Autodesk Inventor part; units mm, degrees
ref_plane "YZ Plane" through (0, 0, 0) normal (1, 0, 0) x (0, 1, 0)
ref_plane "XZ Plane" through (0, 0, 0) normal (0, 1, 0) x (-1, 0, 0)
ref_plane "XY Plane" through (0, 0, 0) normal (0, 0, 1) x (1, 0, 0)
sketch "Sketch1" plane through (0, 0, 0) normal (0, 0, 1) x (1, 0, 0)
  line L0 (-33.82, 21.26) -> (-13.5, 21.26)
  line L1 (-13.5, 21.26) -> (-13.5, 6.02)
  line L2 (-13.5, 6.02) -> (-16.04, 6.02)
  line L3 (-16.04, 6.02) -> (-18.58, 16.18)
  line L4 (-18.58, 16.18) -> (-33.82, 16.18)
  line L5 (-33.82, 16.18) -> (-33.82, 21.26)
  dimension "d0" = 20.32
  dimension "d1" = 15.24
  dimension "d2" = 5.08
  dimension "d3" = 2.54
  dimension "d4" = 15.24
extrude "Extrusion1" add sketch "Sketch1" along normal blind 2.54
ref_plane "Work Plane1" through (0, 0, 1.27) normal (0, 0, 1) x (1, 0, 0)
sketch "Sketch2" plane through (0, 0, 1.27) normal (0, 0, 1) x (1, 0, 0)
  line L0 (-33.82, 18.974) -> (-36.36, 18.974)
  arc A0 (-36.36, 18.974) -> (-35.5534, 12.624) centre (-10.96, 18.974) ccw
  line L1 (-35.5534, 12.624) -> (-33.82, 12.624)
  line L2 (-33.82, 12.624) -> (-33.82, 18.974)
  line L3 (-33.82, 16.18) -> (-33.82, 21.26)
  line L4 (-33.82, 21.26) -> (-13.5, 21.26)
  dimension "d8" = 2.54
  dimension "d9" = 6.35
  dimension "d10" = 25.4
  dimension "d11" = 2.286
revolve "Revolution1" add sketch "Sketch2" angle 360 about axis through (-33.82, 18.974, 1.27) along (-1, 0, 0)
sketch "Sketch3" plane through (0, 0, 1.27) normal (0, 0, 1) x (1, 0, 0)
  line L0 (-16.04, 6.02) -> (-18.58, 6.02)
  line L1 (-18.58, 6.02) -> (-18.58, 18.72)
  line L2 (-18.58, 18.72) -> (-16.04, 18.72)
  line L3 (-16.04, 18.72) -> (-16.04, 6.02)
  line L4 (-13.5, 6.02) -> (-16.04, 6.02)
  dimension "d13" = 12.7
  dimension "d14" = 2.54
extrude "Extrusion2" add sketch "Sketch3" along normal mid plane 1.016
sketch "Sketch4" plane through (-13.5, 6.02, 0) normal (1, 0, 0) x (0, 0, -1)
  line L0 (-2.54, 15.24) -> (-2.54, 0)
  line L1 (0, 15.24) -> (-2.54, 15.24)
  line L2 (-2.54, 0) -> (99.06, 0)
  line L3 (-2.54, 6.35) -> (99.06, 6.35)
  line L4 (99.06, 6.35) -> (99.06, 0)
  dimension "d17" = 6.35
  dimension "d18" = 101.6
extrude "Extrusion3" add sketch "Sketch4" against normal blind 2.54
ref_plane "Work Plane2" through (-13.5, 13.64, 0) normal (0, 1, 0) x (1, 0, 0)
sketch "Sketch5" plane through (-13.5, 13.64, 0) normal (0, 1, 0) x (1, 0, 0)
  circle A0 centre (-1.27, 29.21) radius 2.286
  line L0 (0, 99.06) -> (0, 0)
  line L1 (-20.32, -2.54) -> (0, -2.54)
  dimension "d22" = 4.572
  dimension "d23" = 1.27
  dimension "d24" = 31.75
extrude "Extrusion4" add sketch "Sketch5" against normal blind 8.89
sketch "Sketch6" plane through (-16.04, 12.37, 0) normal (0, 1, 0) x (1, 0, 0)
  arc A0 (0, 27.3092) -> (2.54, 27.3092) centre (1.27, 29.21) ccw
  line L0 (0, 27.3092) -> (0, 0)
  line L1 (2.54, 27.3092) -> (2.54, 0)
  line L2 (1.27, 29.21) -> (-2.54, 29.21)
  line L3 (-2.54, 29.21) -> (-2.54, 27.178)
  line L4 (-2.54, 27.178) -> (1.27, 27.178)
  line L5 (1.27, 27.178) -> (1.27, 29.21)
  line L6 (-2.54, -1.778) -> (-2.54, -0.762)
  dimension "d27" = 2.032
extrude "Extrusion5" add sketch "Sketch6" against normal up to surface (6.35 mm away)
sketch "Sketch7" plane through (-16.04, 6.02, -99.06) normal (0, -1, 0) x (1, 0, 0)
  line L0 (0, 67.9492) -> (0, 0)
  line L1 (2.54, 67.9492) -> (2.54, 0)
  circle A0 centre (1.27, 0) radius 3.81
  circle A1 centre (1.27, 0) radius 1.27 construction
  arc A2 (2.54, 71.7508) -> (-1.016, 69.85) centre (1.27, 69.85) ccw
  dimension "d31" = 7.62
  dimension "d42" = 69.85
extrude "Extrusion6" add sketch "Sketch7" against normal up to surface (6.35 mm away)
sketch "Sketch8" plane through (-14.77, 6.02, -29.21) normal (0, -1, 0) x (1, 0, 0)
  arc A0 (-1.27, -66.2579) -> (1.27, -66.2579) centre (0, -69.85) ccw
hole "Hole1" at (-14.77, 6.02, -99.06) direction (0, 1, 0) diameter 3.81 end through all
sketch "Sketch9" plane through (-13.5, 6.02, 2.54) normal (1, 0, 0) x (0, 0, -1)
  line L0 (29.8492, 6.35) -> (2.54, 6.35)
  line L1 (0, 0) -> (29.8492, 0)
  circle A0 centre (14.8195, 3.175) radius 3.175 construction
  line L2 (0, 15.24) -> (0, 0)
  line L3 (12.7, 4.699) -> (25.4, 4.699)
  line L4 (25.4, 4.699) -> (25.4, 1.651)
  line L5 (25.4, 1.651) -> (12.7, 1.651)
  line L6 (12.7, 1.651) -> (12.7, 4.699)
  circle A1 centre (14.8195, 3.175) radius 1.524 construction
  dimension "d46" = 12.7
  dimension "d47" = 12.7
  dimension "d48" = 3.048
extrude "Extrusion7" cut sketch "Sketch9" against normal blind 1.27
properties part number "lock"
Design review of the part built by this model. Coordinates are the model's own, in mm. A direction names the side the tool comes from. Give positions to 0.01 mm unless a question says otherwise; leave off trailing zeros. Order: outer loops, then holes, each group sorted by start corner. A loop starts at its lowest first (then second) coordinate and runs counter-clockwise, first axis right, second up.
1. Tool access review of faces 4 (the flat face through (-15, 12.37, -69)), 5 (the flat face through (-13.5, 9, -64)), 6 (the flat face through (-15, 6.02, -69)), 7 (the flat face through (-16.04, 9, -13)), 8 (the flat face through (-14.77, 9, -16)): name each direction out of +Z, -Z, +X, -X, +Y, -Y from which nothing blocks a thin tool from reaching the whole face with its end or side.
Solution:
face 4: -Z, +X, -X, +Y
face 5: +X, +Y, -Y
face 6: -Z, +X, -X, -Y
face 7: -X, +Y, -Y
face 8: +X
2. To check wall thickness, follow L1, parallel to X at y = 8.5, z = -99.06 (3 decimals); L2, parallel to Z at x = -14.77, y = 11 (3 decimals); L3, parallel to Y at x = -14.25, z = -21. State the ranges of each line that lie inside material, in increasing order.
Solution:
L1: x = -18.58 to -16.675, -12.865 to -10.96
L2: z = -102.87 to -100.965, -97.155 to 2.54
L3: y = 6.02 to 7.67, 10.72 to 12.37
3. For pin 1 Ø1.3 at (x, y) = (-17, 11.5) entering from -Z; pin 2 Ø1.3 at (x, z) = (-23, 1.5) entering from -Y; pin 3 Ø3 at (y, z) = (8.5, -49) entering from -X, all flat-tipped, find the tip position at first contact; note any pin that passes through.
Solution:
pin 1: stops at z = -102.53
pin 2: stops at y = 16.18
pin 3: stops at x = -16.04
4. Mouldability with a two-part tool opening along Z and no side actions: class faces 1 (the flat face through (-15, 6.02, -14)), 2 (the flat face through (-18, 9, 1.778)), 3 (the flat face through (-18, 9, 0.762)) as +Z half, -Z half, draft (parallel to the pull), parting line (faces both ways), or undercut.
Solution:
face 1: draft
face 2: +Z half
face 3: undercut
5. Add section B-B, the plane x = -29. State the section outline as (y, z) points.
Solution:
outline: (16.18, 0) - (21.26, 0) - (21.26, 2.54) - (16.18, 2.54) - close
6. Add section A-A, the plane z = -99.06. State the section outline as (x, y) points (3 decimals).
Solution:
outline: (-18.58, 6.02) - (-16.675, 6.02) - (-16.675, 12.37) - (-18.58, 12.37) - close; (-12.865, 6.02) - (-10.96, 6.02) - (-10.96, 12.37) - (-12.865, 12.37) - close
